Can you work these out from the model? Positions are in its coordinate system, mm. A direction names the side the tool comes from. Coordinates: 2 decimals unless noted, no trailing zeros. Order: outer loops, then holes, each group sorted by start corner. A loop starts at its lowest first (then second) coordinate and runs counter-clockwise, first axis right, second up. Notation, with made-up numbers: (26.5, 48.5) - (31.5, 48.5) arc R8 ccw to (31.5, 56.5) - close; hole circle Ø4 at (72, -19.5). An arc over 180 degrees is marked (long way). Use a Markdown table: item, result. Add a question column.
(1) I want a section at A-A (z = 55). List the corners of the cut face in (x, y) for me.
(2) For pin 1 Ø4 at (y, z) = (14.5, 52) entering from -X; pin 2 Ø12 at (x, z) = (49.5, 59) entering from +Y; pin 3 Ø12 at (x, z) = (35.5, 66) entering from +Y, each with a flat end and sliding along its axis, tell me the tip position at first contact or that it passes through.
(3) We'd pull the mould along Y, two halves only. Please class faces 3 (the flat face through (23, -2, 41)), 4 (the flat face through (58, 49, 29)), 5 (the flat face through (38, 95, 55)): pulls with the +Y half, pulls with the -Y half, needs draft (parallel to the pull), parting line crosses it, or undercut.
(4) I want a section at C-C (y = 50). List the corners of the cut face in (x, z) for me, and give its area (3 significant figures).
(5) If I drill on L1, parallel to Y at x = 6.5, z = 26.5; L2, parallel to X at y = 49.5, z = 34; L3, parallel to X at y = 23.5, z = 16.5, over which ranges is the centre line in solid material (lowest first)? Write a range as [from, to].
(6) On a 3-axis mill with a long thin cutter (end or side, diameter ignored), from which of +Z, -Z, +X, -X, +Y, -Y can I reach the whole of each face in a straight line? I mean faces 1 (the flat face through (48, 89, 35)), 2 (the cylindrical face through (53.07, 87.153, 34.234)). Say none if no direction works.
(7) I want a section at B-B (x = 56.5). List the corners of the cut face in (y, z) for me.
(8) I want a section at D-D (x = 28). List the corners of the cut face in (y, z) for me, and give its area (3 significant figures).
```python
from build123d import *

# Parameters (mm, degrees)
F0_W     = 2
F0_H     = 50
F1_DEPTH = 2
F2_DEPTH = 100
F3_R     = 4
F3_R_2   = 2
F4_DEPTH = 10
F3_R_3   = 2.064533
F5_DEPTH = 20


with BuildPart() as f1:
    # F0 (on Front) → F1 (new body)
    with BuildSketch(Plane.XZ):
        Polygon((0, 80), (0, 0), (60, 0), (60, 10), (58, 10), (58, 60), (60, 60), (60, 80), align=None)
        with BuildLine():
            Line((26, 17), (26, 63))
            ThreePointArc((26, 63), (28, 65), (30, 63))
            Line((30, 63), (30, 17))
            ThreePointArc((30, 17), (28, 15), (26, 17))
        make_face(mode=Mode.SUBTRACT)
        Polygon((43, 67), (52, 67), (52, 13), (49, 13), (49, 26), (46, 26), (46, 39), (43, 39), align=None, mode=Mode.SUBTRACT)
        with Locations((59, 35)):
            Rectangle(F0_W, F0_H)
    extrude(amount=F1_DEPTH)

    # F0 (on Front) → F2 (join)
    with BuildSketch(Plane.XZ):
        with Locations((59, 35)):
            Rectangle(F0_W, F0_H)
    extrude(amount=-F2_DEPTH)

    # F3 (on face) → F4 (join)
    with BuildSketch(Plane(origin=(58, 0, 0), x_dir=(0, -1, 0), z_dir=(-1, 0, 0))):
        with Locations((-50, 35)):
            Circle(F3_R)
        with Locations((-89, 35)):
            Circle(F3_R_2)
    extrude(amount=F4_DEPTH)

    # F3 (on face) → F5 (join)
    with BuildSketch(Plane(origin=(58, 0, 0), x_dir=(0, -1, 0), z_dir=(-1, 0, 0))):
        with Locations((-95, 55)):
            Circle(F3_R_3)
    extrude(amount=F5_DEPTH)


solid = f1.part
```
Answers follow:
| question | item | result |
|---|---|---|
| 1 | outline | (0, -2) - (26, -2) - (26, 0) - (0, 0) - close; (30, -2) - (43, -2) - (43, 0) - (30, 0) - close; (38, 92.94) - (58, 92.94) - (58, 0) - (52, 0) - (52, -2) - (60, -2) - (60, 100) - (58, 100) - (58, 97.06) - (38, 97.06) - close |
| 2 | pin 1 | stops at x = 58 |
| 2 | pin 2 | stops at y = 97.06 |
| 2 | pin 3 | stops at y = 0 |
| 3 | face 3 | pulls with the -Y half |
| 3 | face 4 | undercut |
| 3 | face 5 | needs draft |
| 4 | outline | (48, 31) - (58, 31) - (58, 10) - (60, 10) - (60, 60) - (58, 60) - (58, 39) - (48, 39) - close |
| 4 | area | 180 mm² |
| 5 | L1 | y = [-2, 0] |
| 5 | L2 | x = [48, 60] |
| 5 | L3 | x = [58, 60] |
| 6 | face 1 | +Z, -Z, -X, +Y, -Y |
| 6 | face 2 | -X |
| 7 | outline | (-2, 0) - (0, 0) - (0, 80) - (-2, 80) - close; circle Ø8 at (50, 35); circle Ø4 at (89, 35); circle Ø4.13 at (95, 55) |
| 8 | outline | (-2, 0) - (0, 0) - (0, 15) - (-2, 15) - close; (-2, 65) - (0, 65) - (0, 80) - (-2, 80) - close |
| 8 | area | 60.0 mm² |
